Build history of the part. All positions in model axes, mm. A direction names the side the tool comes from. Give positions to 0.01 mm unless a question says otherwise; leave off trailing zeros. Write each loop counter-clockwise with the first axis right and the second up, starting at its lowest first coordinate (ties: lowest second). Pieces come first, ordered by that corner, then holes. Notation, with made-up numbers: M 15,-36 L 35,-36 A14 cw 35,-18 Z; hole C -1,4.5 d1. An arc over 180 degrees is marked long. One line per item, written item: value. Start each with the question number.
from build123d import *

# Parameters (mm, degrees)
BOSS_EXTRUDE1_DEPTH  = 3
M3_CLEARANCE_HOLE3_D = 3.4


with BuildPart() as part:
    # Sketch1 → Boss-Extrude1 (new body)
    with BuildSketch(Plane(origin=(0, 0, 0), x_dir=(1, 0, 0), z_dir=(0, 1, 0))):
        with BuildLine():
            Line((-18.384776311, 14.142135624), (-12.727922061, 8.485281374))
            ThreePointArc((-12.727922061, 8.485281374), (-9.213203436, 0), (-12.727922061, -8.485281374))
            Line((-12.727922061, -8.485281374), (-18.384776311, -14.142135624))
            ThreePointArc((-18.384776311, -14.142135624), (-18.384776311, -18.384776311), (-14.142135624, -18.384776311))
            Line((-14.142135624, -18.384776311), (-8.485281374, -12.727922061))
            ThreePointArc((-8.485281374, -12.727922061), (0, -9.213203436), (8.485281374, -12.727922061))
            Line((8.485281374, -12.727922061), (14.142135624, -18.384776311))
            ThreePointArc((14.142135624, -18.384776311), (18.384776311, -18.384776311), (18.384776311, -14.142135624))
            Line((18.384776311, -14.142135624), (12.727922061, -8.485281374))
            ThreePointArc((12.727922061, -8.485281374), (9.213203436, 0), (12.727922061, 8.485281374))
            Line((12.727922061, 8.485281374), (18.384776311, 14.142135624))
            ThreePointArc((18.384776311, 14.142135624), (18.384776311, 18.384776311), (14.142135624, 18.384776311))
            Line((14.142135624, 18.384776311), (8.485281374, 12.727922061))
            ThreePointArc((8.485281374, 12.727922061), (0, 9.213203436), (-8.485281374, 12.727922061))
            Line((-8.485281374, 12.727922061), (-14.142135624, 18.384776311))
            ThreePointArc((-14.142135624, 18.384776311), (-18.384776311, 18.384776311), (-18.384776311, 14.142135624))
        make_face()
    extrude(amount=BOSS_EXTRUDE1_DEPTH)

    # M3 Clearance Hole3 (through all)
    with Locations(Plane(origin=(0, 3, 0), x_dir=(1, 0, 0), z_dir=(0, 1, 0))):
        with Locations((-16.379512961, -16.263455967), (-10.606601718, -10.606601718), (16.263455967, -16.263455967), (10.606601718, -10.606601718), (16.147398973, 16.263455967), (10.606601718, 10.606601718), (-10.606601718, 10.606601718), (-16.263455967, 16.263455967)):
            Hole(M3_CLEARANCE_HOLE3_D / 2)


solid = part.part
1) Band-saw the part on C-C (y = 1.2). Count the separate pieces of the cut face and the enclosed holes in it, then the cut area to 3 significant figures.
2) Probe line 1 along X through (y, z) = (1.75, 11); line 2 along X through (y, z) = (1, 11.5). List the from-to ranges inside material, lowest first. Write a range as from..to.
3) Tool access for faces 1 (the face through (-15.517, 1.479, 11.274)), 2 (the face through (-11.274, 1.479, -15.517)), 3 (the face through (15.517, 1.479, -11.274)), 4 (the face through (0, 0, 0)): list every direction of +Z, -Z, +X, -X, +Y, -Y with a clear straight run to the whole face (end or side of a thin tool).
4) Band-saw the part on B-B (z = 13.5). List the corners of the cut face in (x, y), then the cut area to 3 significant figures.
5) Mould opens along Z. For faces 5 (the face through (0, 3, 0)), 6 (the face through (9.214, 1.479, 0.132)), 7 (the face through (-11.353, 1.479, 15.596)), 8 (the face through (11.353, 1.479, -15.596)) say: released by +Z, released by -Z, zero draft, split by the parting line, or undercut.
6) Band-saw the part on D-D (z = -15). List the corners of the cut face in (x, y).
7) Drop flat-ended pins along their axis: P1, Ø4, axis at x = 16.26, z = 16.26, coming from the +Y side; P2, Ø3, axis at x = 16.15, z = -16.26, coming from the -Y side. Give the stop position or say it passes through.
8) Band-saw the part on A-A (x = -10). List the corners of the cut face in (y, z), then the cut area to 3 significant figures.
Model answer:
1. separate pieces: 1
1. enclosed holes: 8
1. area: 624 mm²
2. line 1: x = -15.24..-12.26, -8.95..-6.3, 6.3..8.95, 12.26..15.24
2. line 2: x = -15.74..-12.05, -9.16..-7.05, 7.05..9.16, 12.05..15.74
3. face 1: -X, +Y, -Y
3. face 2: -Z, +Y, -Y
3. face 3: +X, +Y, -Y
3. face 4: +Z, -Z, +X, -X, -Y
4. outline: M -17.74,0 L -9.26,0 L -9.26,3 L -17.74,3 Z; M 9.26,0 L 17.74,0 L 17.74,3 L 9.26,3 Z
4. area: 50.9 mm²
5. face 5: zero draft
5. face 6: undercut
5. face 7: released by +Z
5. face 8: released by -Z
6. outline: M -18.98,0 L -17.4,0 L -17.4,3 L -18.98,3 Z; M -15.13,0 L -10.76,0 L -10.76,3 L -15.13,3 Z; M 10.76,0 L 15.01,0 L 15.01,3 L 10.76,3 Z; M 17.28,0 L 18.98,0 L 18.98,3 L 17.28,3 Z
7. P1: stops at y = 3
7. P2: passes through
8. outline: M 0,-14.24 L 3,-14.24 L 3,-12.19 L 0,-12.19 Z; M 0,-9.02 L 3,-9.02 L 3,-4.27 L 0,-4.27 Z; M 0,4.27 L 3,4.27 L 3,9.02 L 0,9.02 Z; M 0,12.19 L 3,12.19 L 3,14.24 L 0,14.24 Z
8. area: 40.8 mm²
